```python
from build123d import *

# Parameters (mm, degrees)
F0_W     = 571.5
F0_H     = 279.4
F1_DEPTH = 4.699
F3_DEPTH = 4.7
F4_R     = 4.7625
F5_DEPTH = 4.7


with BuildPart() as f1:
    # F0 (on Front) → F1 (new body)
    with BuildSketch(Plane.XZ):
        Rectangle(F0_W, F0_H)
    extrude(amount=F1_DEPTH)

    # F2 (on face) → F3 (cut, through all)
    with BuildSketch(Plane.XZ.offset(4.699)):
        with BuildLine():
            Line((247.65, 114.3), (-247.65, 114.3))
            ThreePointArc((-247.65, 114.3), (-256.630256, 110.580256), (-260.35, 101.6))
            Line((-260.35, 101.6), (-260.35, -101.6))
            ThreePointArc((-260.35, -101.6), (-256.630256, -110.580256), (-247.65, -114.3))
            Line((-247.65, -114.3), (247.65, -114.3))
            ThreePointArc((247.65, -114.3), (256.630256, -110.580256), (260.35, -101.6))
            Line((260.35, -101.6), (260.35, 101.6))
            ThreePointArc((260.35, 101.6), (256.630256, 110.580256), (247.65, 114.3))
        make_face()
    extrude(amount=-F3_DEPTH, mode=Mode.SUBTRACT)

    # F4 (on face) → F5 (cut, through all)
    with BuildSketch(Plane.XZ.offset(4.699)):
        with Locations((-266.7, -120.65)):
            Circle(F4_R)
        with Locations((0, -120.65)):
            Circle(F4_R)
        with Locations((266.7, -120.65)):
            Circle(F4_R)
        with Locations((266.7, 120.65)):
            Circle(F4_R)
        with Locations((0, 120.65)):
            Circle(F4_R)
        with Locations((-266.7, 120.65)):
            Circle(F4_R)
    extrude(amount=-F5_DEPTH, mode=Mode.SUBTRACT)


solid = f1.part
```
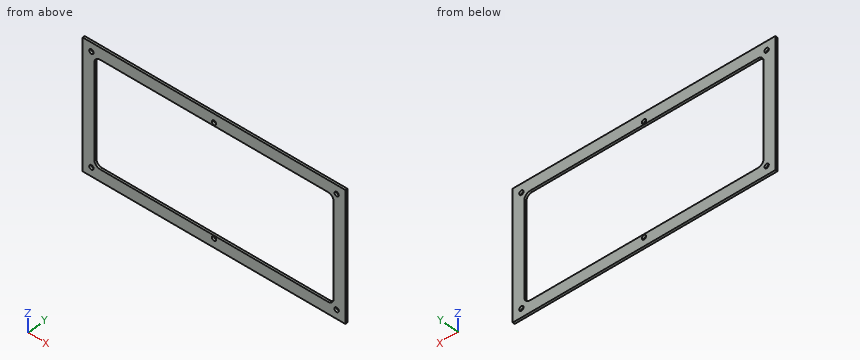
Input: part model. Units: mm. Frame: model coordinates. Round coordinates to 2 decimals unless told otherwise and drop trailing zeros. Loops run counter-clockwise (first coordinate to the right, second up) from the corner with the lowest first, then second, coordinate; pieces in that order, holes last. Notation, with made-up numbers: M 59.25,-23 L 88.25,-23 A21 cw 88.25,3 Z; hole C 12,-13.5 d4. An arc over 180 degrees is marked long. Answer in a Markdown table with one row per item. Add a question column.
1. Section B-B (z = -63). Output: boundary loops of the cut face in (x, y).
2. Contact query for a flat-ended pin moving along its axis: pin 1 (15 mm diameter, centred on x = 0, z = -120.65, fed in from -Y). Output: stop coordinate, or through.
3. Section A-A (x = 76). Output: boundary loops of the cut face in (y, z), and give its area (3 significant figures).
4. Section C-C (y = -1.95). Give the number of separate pieces and of enclosed holes in the cut face, and give its area (3 significant figures).
5. Ray query, probe 1 along Z at (x, y) = (-266.7, -1.65); probe 2 along Z at (x, y) = (0, -1.8); probe 3 along Z at (x, y) = (-32, -3.45). Return the intervals inside material, ascending.
Values follow:
| question | item | result |
|---|---|---|
| 1 | outline | M -285.75,-4.7 L -260.35,-4.7 L -260.35,0 L -285.75,0 Z; M 260.35,-4.7 L 285.75,-4.7 L 285.75,0 L 260.35,0 Z |
| 2 | pin 1 | y = -4.7 |
| 3 | outline | M -4.7,-139.7 L 0,-139.7 L 0,-114.3 L -4.7,-114.3 Z; M -4.7,114.3 L 0,114.3 L 0,139.7 L -4.7,139.7 Z |
| 3 | area | 239 mm^2 |
| 4 | separate pieces | 1 |
| 4 | enclosed holes | 7 |
| 4 | area | 40,400 mm^2 |
| 5 | probe 1 | -139.7 to -125.41, -115.89 to 115.89, 125.41 to 139.7 |
| 5 | probe 2 | -139.7 to -125.41, -115.89 to -114.3, 114.3 to 115.89, 125.41 to 139.7 |
| 5 | probe 3 | -139.7 to -114.3, 114.3 to 139.7 |
